For this review, take the finished solid that the model builds, in its own axes (mm). A direction names the side the tool comes from. Round coordinates to 2 decimals unless told otherwise and drop trailing zeros. Write each loop counter-clockwise with the first axis right and the second up, starting at its lowest first coordinate (ties: lowest second). Pieces come first, ordered by that corner, then holes. Notation, with made-up numbers: (57, 33.25) -> (112, 33.25) arc R29 ccw to (112, 65.25) -> close; hole circle Ø2 at (-37.5, 81.5). An arc over 180 degrees is marked (long way). Answer in a Markdown table with one row per item.
from build123d import *

# Parameters (mm, degrees)
SKETCH001_R      = 3.96875
EXTRUDE001_DEPTH = 76.2
EXTRUDE_DEPTH    = 6
FILLET_R         = 1
FILLET001_R      = 1


with BuildPart() as extrude001:
    # Sketch001 (on Face8 of Extrude) → Extrude001 (new body)
    with BuildSketch(Plane.XY.offset(6)):
        Circle(SKETCH001_R)
    extrude(amount=EXTRUDE001_DEPTH)


with BuildPart() as fillet001:
    # Sketch → Extrude (new body)
    with BuildSketch(Plane.XY):
        Polygon((0, -7.505553), (6.5, -3.752777), (6.5, 3.752777), (0, 7.505553), (-6.5, 3.752777), (-6.5, -3.752777), align=None)
    extrude(amount=EXTRUDE_DEPTH)

    # Fusion: union Extrude001
    add(extrude001.part)

    # Fillet
    fillet_edges = [fillet001.edges().sort_by_distance(p)[0] for p in [
        (-3.96875, 0, 82.2),
    ]]
    fillet(fillet_edges, radius=FILLET_R)

    # Fillet001
    fillet001_edges = [fillet001.edges().sort_by_distance(p)[0] for p in [
        (3.25, -5.629165, 0),
        (-3.25, -5.629165, 0),
        (6.5, 0, 0),
        (-6.5, 0, 0),
        (3.25, 5.629165, 0),
        (-3.25, 5.629165, 0),
    ]]
    fillet(fillet001_edges, radius=FILLET001_R)


solid = fillet001.part
1) For line 1 (Z direction, x = -0.75, y = -5.5); line 2 (Y direction, x = -3.5, z = 5); line 3 (Y direction, x = -3.25, z = 70), list the stretches that pass through material, from the lowest coordinate up. Write a range as [from, to].
Solved:
| item | result |
|---|---|
| line 1 | [0, 6] |
| line 2 | [-5.48, 5.48] |
| line 3 | [-2.28, 2.28] |
2) Consider section B-B on z = 31. State the section outline as (x, y) points, then the cut area to 3 significant figures.
Solved:
| item | result |
|---|---|
| outline | circle Ø7.94 at (0, 0) |
| area | 49.5 mm² |
3) Consider section A-A on y = 0. State the section outline as (x, z) points, then the cut area to 3 significant figures.
Solved:
| item | result |
|---|---|
| outline | (-6.5, 1) arc R1 ccw to (-5.5, 0) -> (5.5, 0) arc R1 ccw to (6.5, 1) -> (6.5, 6) -> (3.97, 6) -> (3.97, 81.2) arc R1 ccw to (2.97, 82.2) -> (-2.97, 82.2) arc R1 ccw to (-3.97, 81.2) -> (-3.97, 6) -> (-6.5, 6) -> close |
| area | 682 mm² |
4) Clearance check with flat-ended pins moving along their axes: pin 1 Ø6 at (x, z) = (-1.5, 13.5) entering from +Y; pin 2 Ø1.5 at (x, y) = (-2.5, -3.5) entering from +Z; pin 3 Ø1 at (x, y) = (-3.5, -1.5) entering from +Z. State where each tip first meets the part, or that it passes through.
Solved:
| item | result |
|---|---|
| pin 1 | y = 3.97 |
| pin 2 | z = 82.01 |
| pin 3 | z = 82.14 |
5) For faces 1 (the flat face through (3.2, -5.66, 3.46)), 2 (the flat face through (-3, -3, 6)), list the 3-axis set-ups (+Z, -Z, +X, -X, +Y, -Y) from which the entire face can be reached by the end or side of a thin tool; tool diameter is ignored.
Solved:
| item | result |
|---|---|
| face 1 | +Z, -Z, +X, -Y |
| face 2 | +Z |
